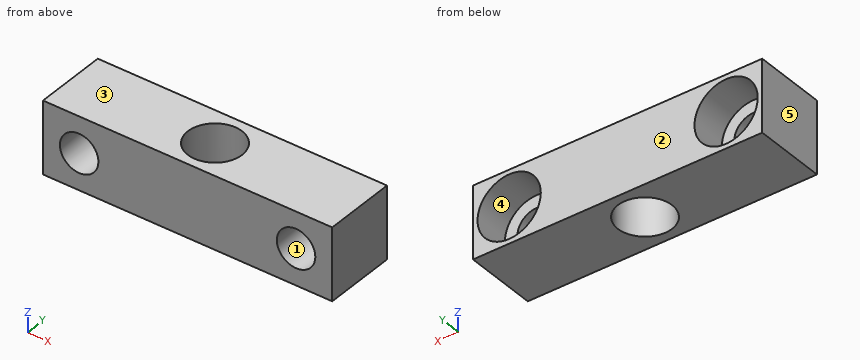
from build123d import *

# Parameters (mm, degrees)
SKETCH1_W                                        = 50.8
SKETCH1_H                                        = 12.7
EXTRUDE1_DEPTH                                   = 12.7
SKETCH3_R                                        = 4.7625
CUT_EXTRUDE2_DEPTH                               = 32.108519733
CBORE_FOR_1_4_SOCKET_HEAD_CAP_SCREW1_D           = 6.7564
CBORE_FOR_1_4_SOCKET_HEAD_CAP_SCREW1_CBORE_D     = 11.1125
CBORE_FOR_1_4_SOCKET_HEAD_CAP_SCREW1_CBORE_DEPTH = 6.35


with BuildPart() as part:
    # Sketch1 → Extrude1 (new body)
    with BuildSketch(Plane(origin=(0, 0, 0), x_dir=(1, 0, 0), z_dir=(0, 1, 0))):
        Rectangle(SKETCH1_W, SKETCH1_H)
    extrude(amount=EXTRUDE1_DEPTH)

    # Sketch3 → Cut-Extrude2 (cut, through all)
    with BuildSketch(Plane.XY.offset(6.35)):
        with Locations((0, 6.35)):
            Circle(SKETCH3_R)
    extrude(amount=-CUT_EXTRUDE2_DEPTH, mode=Mode.SUBTRACT)

    # CBORE for 1/4 Socket Head Cap Screw1 (through all)
    with Locations(Plane(origin=(0, 12.7, 0), x_dir=(-1, 0, 0), z_dir=(0, 1, 0))):
        with Locations((-19.05, 0), (19.05, 0)):
            CounterBoreHole(CBORE_FOR_1_4_SOCKET_HEAD_CAP_SCREW1_D / 2, CBORE_FOR_1_4_SOCKET_HEAD_CAP_SCREW1_CBORE_D / 2, CBORE_FOR_1_4_SOCKET_HEAD_CAP_SCREW1_CBORE_DEPTH)


solid = part.part
CAD build for the part. Positions are in the model's coordinates, mm. Face numbers are marked on the shaded views. A direction names the side the tool comes from. Give positions to 0.01 mm unless a question says otherwise; leave off trailing zeros. Loops run counter-clockwise (first coordinate to the right, second up) from the corner with the lowest first, then second, coordinate; pieces in that order, holes last. Notation, with made-up numbers: M 21,36.5 L 74,36.5 A15 ccw 74,65.5 Z; hole C 48.5,80 d10. An arc over 180 degrees is marked long. Answer in a Markdown table with one row per item. Add a question column.
Item 1: Probe probe 1 along X at (y, z) = (4.5, -2.5); probe 2 along Y at (x, z) = (0, 3); probe 3 along X at (y, z) = (3.25, 0.75). List the from-to ranges inside material, lowest first.
Item 2: Drop a flat-ended pin along its axis: P1, Ø5.5, axis at x = 19.05, z = 0, coming from the -Y side. Give the stop position or say it passes through.
Item 3: Tool access for the marked faces 4 and 5: list every direction of +Z, -Z, +X, -X, +Y, -Y with a clear straight run to the whole face (end or side of a thin tool).
Item 4: Band-saw the part on D-D on x = 0. Give the cut face in (y, z).
Item 5: Band-saw the part on C-C on y = 7.25. Give the cut face in (x, z), then the cut area to 3 significant figures.
Item 6: Band-saw the part on A-A on z = 0. Give the number of separate pieces and of enclosed holes in the cut face, then the cut area to 3 significant figures.
Item 7: Mould opens along Z. For the marked faces 1, 2 and 3 say: +Z half, -Z half, draft (parallel to the pull), parting line (faces both ways), or undercut.
Item 8: Band-saw the part on B-B on x = 19.05. Give the cut face in (y, z), then the cut area to 3 significant figures.
Reply:
| question | item | result |
|---|---|---|
| 1 | probe 1 | x = -25.4 to -21.32, -16.78 to -4.39, 4.39 to 16.78, 21.32 to 25.4 |
| 1 | probe 2 | y = 0 to 1.59, 11.11 to 12.7 |
| 1 | probe 3 | x = -25.4 to -22.34, -15.76 to -3.62, 3.62 to 15.76, 22.34 to 25.4 |
| 2 | P1 | passes through |
| 3 | face 4 | +Y |
| 3 | face 5 | +Z, -Z, -X, +Y, -Y |
| 4 | outline | M 0,-6.35 L 1.59,-6.35 L 1.59,6.35 L 0,6.35 Z; M 11.11,-6.35 L 12.7,-6.35 L 12.7,6.35 L 11.11,6.35 Z |
| 5 | outline | M -25.4,-6.35 L -4.68,-6.35 L -4.68,6.35 L -25.4,6.35 Z; M 4.68,-6.35 L 25.4,-6.35 L 25.4,6.35 L 4.68,6.35 Z; hole C -19.05,0 d11.11; hole C 19.05,0 d11.11 |
| 5 | area | 332 mm^2 |
| 6 | separate pieces | 3 |
| 6 | enclosed holes | 1 |
| 6 | area | 347 mm^2 |
| 7 | face 1 | undercut |
| 7 | face 2 | draft |
| 7 | face 3 | +Z half |
| 8 | outline | M 0,-6.35 L 12.7,-6.35 L 12.7,-5.56 L 6.35,-5.56 L 6.35,-3.38 L 0,-3.38 Z; M 0,3.38 L 6.35,3.38 L 6.35,5.56 L 12.7,5.56 L 12.7,6.35 L 0,6.35 Z |
| 8 | area | 47.8 mm^2 |
